from build123d import *

# Parameters (mm, degrees)
SKETCH_1_W      = 20
SKETCH_1_H      = 15
EXTRUDE_1_DEPTH = 3
SKETCH_2_W      = 8
SKETCH_2_H      = 6
EXTRUDE_2_DEPTH = 0.5
FILLET_1_R      = 1
FILLET_2_R      = 1.1
FILLET_3_R      = 0.1


with BuildPart() as part:
    # 草图1 → 凸台-拉伸1 (new body)
    with BuildSketch(Plane(origin=(0, 0, 0), x_dir=(1, 0, 0), z_dir=(0, 1, 0))):
        Rectangle(SKETCH_1_W, SKETCH_1_H)
    extrude(amount=EXTRUDE_1_DEPTH)

    # 草图2 → 凸台-拉伸2 (add)
    with BuildSketch(Plane(origin=(0, 3, 0), x_dir=(1, 0, 0), z_dir=(0, 1, 0))):
        Rectangle(SKETCH_2_W, SKETCH_2_H)
    extrude(amount=EXTRUDE_2_DEPTH)

    # 圆角1
    fillet_1_edges = [part.edges().sort_by_distance(p)[0] for p in [
        (-4, 3.25, -3),
        (-4, 3.25, 3),
        (4, 3.25, 3),
        (4, 3.25, -3),
    ]]
    fillet(fillet_1_edges, radius=FILLET_1_R)

    # 圆角2
    # the kernel refuses this fillet: 1.1 mm, written as the material it adds along each edge
    with BuildSketch(Plane(origin=(3, 3, 2), x_dir=(0, 0, 1), z_dir=(-1, 0, 0))) as fillet_2_piece_1:
        with BuildLine():
            CenterArc((1.921954446, 1.1), FILLET_2_R, 213.055731151, 56.944268849)
            Line((1, 0.5), (0.981560911, 0.488))
            ThreePointArc((0.981560911, 0.488), (0.978, 0.25), (0.978, 0))
            Line((0.978, 0), (1, -0.022))
            Line((1, -0.022), (1.921954446, -0.022))
            Line((1.921954446, -0.022), (1.921954446, 0))
        make_face()
    revolve(axis=Axis((3, 3, 2), (0, 1, 0)), revolution_arc=90)
    with BuildSketch(Plane(origin=(-3, 3, 3), x_dir=(0, 0, 1), z_dir=(1, 0, 0)), Plane(origin=(3, 3, -3), x_dir=(0, 0, -1), z_dir=(-1, 0, 0))) as fillet_2_piece_2:
        with BuildLine():
            CenterArc((0.921954446, -1.1), FILLET_2_R, 90, 56.944268849)
            Line((0, -0.5), (-0.018439089, -0.488))
            ThreePointArc((-0.018439089, -0.488), (-0.022, -0.25), (-0.022, 0))
            Line((-0.022, 0), (0, 0.022))
            Line((0, 0.022), (0.921954446, 0.022))
            Line((0.921954446, 0.022), (0.921954446, 0))
        make_face()
    extrude(amount=6)
    with BuildSketch(Plane(origin=(-3, 3, 2), x_dir=(-1, 0, 0), z_dir=(0, 0, -1))) as fillet_2_piece_3:
        with BuildLine():
            CenterArc((1.921954446, 1.1), FILLET_2_R, 213.055731151, 56.944268849)
            Line((1, 0.5), (0.981560911, 0.488))
            ThreePointArc((0.981560911, 0.488), (0.978, 0.25), (0.978, 0))
            Line((0.978, 0), (1, -0.022))
            Line((1, -0.022), (1.921954446, -0.022))
            Line((1.921954446, -0.022), (1.921954446, 0))
        make_face()
    revolve(axis=Axis((-3, 3, 2), (0, 1, 0)), revolution_arc=90)
    with BuildSketch(Plane(origin=(-4, 3, -2), x_dir=(-1, 0, 0), z_dir=(0, 0, 1)), Plane(origin=(4, 3, 2), x_dir=(1, 0, 0), z_dir=(0, 0, -1))) as fillet_2_piece_4:
        with BuildLine():
            CenterArc((0.921954446, -1.1), FILLET_2_R, 90, 56.944268849)
            Line((0, -0.5), (-0.018439089, -0.488))
            ThreePointArc((-0.018439089, -0.488), (-0.022, -0.25), (-0.022, 0))
            Line((-0.022, 0), (0, 0.022))
            Line((0, 0.022), (0.921954446, 0.022))
            Line((0.921954446, 0.022), (0.921954446, 0))
        make_face()
    extrude(amount=4)
    with BuildSketch(Plane(origin=(-3, 3, -2), x_dir=(0, 0, -1), z_dir=(1, 0, 0))) as fillet_2_piece_5:
        with BuildLine():
            CenterArc((1.921954446, 1.1), FILLET_2_R, 213.055731151, 56.944268849)
            Line((1, 0.5), (0.981560911, 0.488))
            ThreePointArc((0.981560911, 0.488), (0.978, 0.25), (0.978, 0))
            Line((0.978, 0), (1, -0.022))
            Line((1, -0.022), (1.921954446, -0.022))
            Line((1.921954446, -0.022), (1.921954446, 0))
        make_face()
    revolve(axis=Axis((-3, 3, -2), (0, 1, 0)), revolution_arc=90)
    with BuildSketch(Plane(origin=(3, 3, -2), x_dir=(0, 0, -1), z_dir=(-1, 0, 0))) as fillet_2_piece_6:
        with BuildLine():
            CenterArc((1.921954446, -1.1), FILLET_2_R, 90, 56.944268849)
            Line((1, -0.5), (0.981560911, -0.488))
            ThreePointArc((0.981560911, -0.488), (0.978, -0.25), (0.978, 0))
            Line((0.978, 0), (1, 0.022))
            Line((1, 0.022), (1.921954446, 0.022))
            Line((1.921954446, 0.022), (1.921954446, 0))
        make_face()
    revolve(axis=Axis((3, 3, -2), (0, -1, 0)), revolution_arc=90)

    # 圆角3
    fillet_3_edges = [part.edges().sort_by_distance(p)[0] for p in [
        (-4, 3.5, 0),
        (0, 3.5, -3),
        (0, 3.5, 3),
        (4, 3.5, 0),
        (-3.707106781, 3.5, 2.707106781),
        (3.707106781, 3.5, 2.707106781),
        (3.707106781, 3.5, -2.707106781),
        (-3.707106781, 3.5, -2.707106781),
    ]]
    fillet(fillet_3_edges, radius=FILLET_3_R)


solid = part.part
The model under review builds one solid part; all positions refer to its coordinate system, in mm. A direction names the side the tool comes from. Round coordinates to 2 decimals unless told otherwise and drop trailing zeros. Write each loop counter-clockwise with the first axis right and the second up, starting at its lowest first coordinate (ties: lowest second). Pieces come first, ordered by that corner, then holes. Notation, with made-up numbers: (-22.5, 9) - (2.5, 9) arc R9 ccw to (2.5, 20) - close; hole circle Ø9 at (7.5, -18). An arc over 180 degrees is marked (long way). One line per item, written item: value. Start each with the question number.
1. Consider section B-B on x = -0.25. Write out the cut boundary in (y, z), and give its area (3 significant figures).
2. Consider section A-A on z = 0.5. Write out the cut boundary in (x, y), and give its area (3 significant figures).
3. Consider section D-D on x = 6.5. Write out the cut boundary in (y, z), and give its area (3 significant figures).
4. To check wall thickness, follow L1, parallel to Y at x = -5.5, z = -2.25; L2, parallel to Y at x = 1.25, z = 3. State the ranges of each line that lie inside material, in increasing order. Write a range as from..to.
5. Consider section C-C on z = 4.25. Write out the cut boundary in (x, y), and give its area (3 significant figures).
6. Machinability: for faces 1 (the face through (0, 3, -5)), 2 (the face through (10, 1, 0)), which of the approach directions +Z, -Z, +X, -X, +Y, -Y give a long, thin tool a straight path to every point of the face, cutting with its end or side? Answer none if there is none.
7. Clearance check with a flat-ended pin moving along its axis: P1, Ø1, axis at x = -1, z = 5, coming from the +Y side. State where the tip first meets the part, or that it passes through.
Checks:
1. outline: (0, -7.5) - (3, -7.5) - (3, -3.92) arc R1.1 cw to (3.46, -3.03) arc R0.1 ccw to (3.5, -2.95) - (3.5, 2.95) arc R0.1 ccw to (3.46, 3.03) arc R1.1 cw to (3, 3.92) - (3, 7.5) - (0, 7.5) - close
1. area: 48.3 mm^2
2. outline: (-10, 0) - (10, 0) - (10, 3) - (4.92, 3) arc R1.1 cw to (4.03, 3.46) arc R0.1 ccw to (3.95, 3.5) - (-3.95, 3.5) arc R0.1 ccw to (-4.03, 3.46) arc R1.1 cw to (-4.92, 3) - (-10, 3) - close
2. area: 64.3 mm^2
3. outline: (0, -7.5) - (3, -7.5) - (3, 7.5) - (0, 7.5) - close
3. area: 45.0 mm^2
4. L1: y = 0..3
4. L2: y = 0..3.48
5. outline: (-10, 0) - (10, 0) - (10, 3) - (-10, 3) - close
5. area: 60.0 mm^2
6. face 1: +Y
6. face 2: +Z, -Z, +X, +Y, -Y
7. P1: stops at y = 3
